Model file for the job. Use its own axes, mm. A direction names the side the tool comes from. Give positions to 0.01 mm unless a question says otherwise; leave off trailing zeros. Loops run counter-clockwise (first coordinate to the right, second up) from the corner with the lowest first, then second, coordinate; pieces in that order, holes last. Notation, with made-up numbers: M 8.25,47.5 L 34.25,47.5 A26 ccw 34.25,77.5 Z; hole C 21,-20 d11. An arc over 180 degrees is marked long. Use CSV: the item, a comma, the result in double quotes. Start each with the question number.
(1) Tool access for faces 4 (the face through (-2.17, 41.16, -9.76)), 5 (the face through (7.371, 57.541, 2.321)), 6 (the face through (-2, 77, 0)), 7 (the face through (3.1, 18, 10.2)): list every direction of +Z, -Z, +X, -X, +Y, -Y with a clear straight run to the whole face (end or side of a thin tool).
(2) Two-plate mould, pull along Z, no slides. Class faces 1 (the face through (9.443, 70.829, 2.974)), 2 (the face through (-0.945, 75.166, -0.724)), 3 (the face through (1, 29.3, -12)): pulls with the +Z half, pulls with the -Z half, needs draft (parallel to the pull), parting line crosses it, or undercut.
(3) Wall check: line 1 along Z through (x, y) = (0, 74.5); line 2 along Y through (x, z) = (-9, -10.25); line 3 along X through (y, z) = (6, 5.5). Give the ranges that are in metal, low to high. Write a range as from..to.
(4) Slice it at B-B on y = 13.5. List the corners of the cut face in (x, z).
(5) Slice it at A-A on y = 23. List the corners of the cut face in (x, z).
(6) Flat gauge pins, fed straight in: P1, Ø10, axis at y = 26, z = -9, coming from the +X side; P2, Ø2, axis at x = 5, y = 20, coming from the +Z side; P3, Ø5, axis at x = -6.5, y = 49, coming from the -Z side. Where does each tip first touch, or does it go through?
```python
from build123d import *

# Parameters (mm, degrees)
FURO_DE_DI_METRO_3_32_0_09375_2_D           = 2.38125
FURO_DE_DI_METRO_3_32_0_09375_2_DEPTH       = 3
FURO_DE_DI_METRO_3_32_0_09375_2_CSINK_D     = 3.65125
FURO_DE_DI_METRO_3_32_0_09375_2_CSINK_ANGLE = 90
FURO_DE_DI_METRO_3_32_0_09375_2_TIP         = 0.715399675
ESBO_O10_OUTSIDE_W                          = 49.582
ESBO_O10_OUTSIDE_H                          = 49.582
ESBO_O10_OUTSIDE_R                          = 7.5
CORTE_EXTRUS_O2_DEPTH                       = 18
FILETE1_R                                   = 3


with BuildPart() as part:
    # Esboço1 → Revolução1 (revolve)
    with BuildSketch(Plane.XY):
        with BuildLine():
            Line((0, 77), (8.9, 77))
            Line((8.9, 77), (9.9, 76))
            Line((9.9, 76), (9.9, 65.8))
            Line((9.9, 65.8), (10, 65.8))
            Line((10, 65.8), (10, 59.8))
            Line((10, 59.8), (9.5, 59.3))
            Line((9.5, 59.3), (8.516386133, 59.3))
            ThreePointArc((8.516386133, 59.3), (7.697234088, 58.873576436), (7.576693512, 57.957979857))
            Line((7.576693512, 57.957979857), (10, 51.3))
            Line((10, 51.3), (10, 31.3))
            Line((10, 31.3), (9.732050808, 30.3))
            ThreePointArc((9.732050808, 30.3), (10.029032337, 29.297868418), (11.05681259, 29.107780314))
            Line((11.05681259, 29.107780314), (11.55681259, 29.3))
            Line((11.55681259, 29.3), (14.5, 29.3))
            Line((14.5, 29.3), (15, 28.8))
            Line((15, 28.8), (15, 0))
            Line((15, 0), (0, 0))
            Line((0, 0), (0, 77))
        make_face()
    revolve(axis=Axis((0, 77, 0), (0, -1, 0)))

    # Furo de diâmetro 3/32 (0.09375)2
    with Locations(Plane(origin=(0, 77, 0), x_dir=(-1, 0, 0), z_dir=(0, 1, 0))):
        with Locations((0, 0)):
            CounterSinkHole(FURO_DE_DI_METRO_3_32_0_09375_2_D / 2, FURO_DE_DI_METRO_3_32_0_09375_2_CSINK_D / 2, depth=FURO_DE_DI_METRO_3_32_0_09375_2_DEPTH, counter_sink_angle=FURO_DE_DI_METRO_3_32_0_09375_2_CSINK_ANGLE)
            with Locations((0, 0, -(FURO_DE_DI_METRO_3_32_0_09375_2_DEPTH + FURO_DE_DI_METRO_3_32_0_09375_2_TIP / 2))):  # 118° drill point
                Cone(0, FURO_DE_DI_METRO_3_32_0_09375_2_D / 2, FURO_DE_DI_METRO_3_32_0_09375_2_TIP, mode=Mode.SUBTRACT)

    # Esboço10 outside → Corte-extrusão2 (cut)
    with BuildSketch(Plane.XZ):
        Rectangle(ESBO_O10_OUTSIDE_W, ESBO_O10_OUTSIDE_H)
        Circle(ESBO_O10_OUTSIDE_R, mode=Mode.SUBTRACT)
    extrude(amount=-CORTE_EXTRUS_O2_DEPTH, mode=Mode.SUBTRACT)

    # Filete1
    filete1_edges = [part.edges().sort_by_distance(p)[0] for p in [
        (-7.5, 18, 0),
    ]]
    fillet(filete1_edges, radius=FILETE1_R)


solid = part.part
```
Reply:
1,face 4,"+Y"
1,face 5,"none"
1,face 6,"+Z, -Z, +X, -X, +Y"
1,face 7,"-Y"
2,face 1,"parting line crosses it"
2,face 2,"undercut"
2,face 3,"needs draft"
3,line 1,"z = -9.9..-1.19, 1.19..9.9"
3,line 2,"y = 18..29.3"
3,line 3,"x = -5.1..5.1"
4,outline,"C 0,0 d15"
5,outline,"C 0,0 d30"
6,P1,"stops at x = 14.46"
6,P2,"stops at z = 14.46"
6,P3,"stops at z = -9.17"
